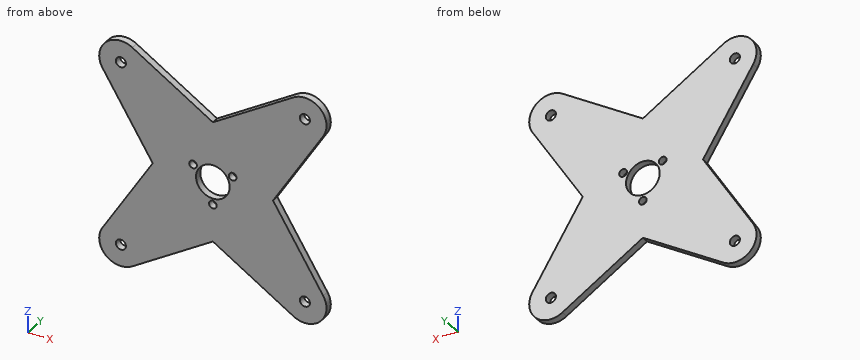
```python
from build123d import *

# Parameters (mm, degrees)
SKETCH_1_R          = 2.1
EXTRUDE_1_DEPTH     = 3
SKETCH_2_R          = 7
SKETCH_2_R_2        = 1.6
CUT_EXTRUDE_1_DEPTH = 10


with BuildPart() as part:
    # 草图1 → 凸台-拉伸1 (new body)
    with BuildSketch(Plane(origin=(0, 0, 0), x_dir=(1, 0, 0), z_dir=(0, 1, 0))):
        with BuildLine():
            Line((-45.88639118, 33.487067107), (-25, 0))
            Line((-25, 0), (-45.88639118, -33.487067107))
            ThreePointArc((-45.88639118, -33.487067107), (-44.613961031, -44.613961031), (-33.487067107, -45.88639118))
            Line((-33.487067107, -45.88639118), (0, -25))
            Line((0, -25), (33.487067107, -45.88639118))
            ThreePointArc((33.487067107, -45.88639118), (44.613961031, -44.613961031), (45.88639118, -33.487067107))
            Line((45.88639118, -33.487067107), (25, 0))
            Line((25, 0), (45.88639118, 33.487067107))
            ThreePointArc((45.88639118, 33.487067107), (44.613961031, 44.613961031), (33.487067107, 45.88639118))
            Line((33.487067107, 45.88639118), (0, 25))
            Line((0, 25), (-33.487067107, 45.88639118))
            ThreePointArc((-33.487067107, 45.88639118), (-44.613961031, 44.613961031), (-45.88639118, 33.487067107))
        make_face()
        with Locations(Location((38.25, 38.25, 0), (0, 0, 270))):
            Circle(SKETCH_1_R, mode=Mode.SUBTRACT)
        with Locations(Location((-38.25, -38.25, 0), (0, 0, 270))):
            Circle(SKETCH_1_R, mode=Mode.SUBTRACT)
        with Locations(Location((38.25, -38.25, 0), (0, 0, 270))):
            Circle(SKETCH_1_R, mode=Mode.SUBTRACT)
        with Locations(Location((-38.25, 38.25, 0), (0, 0, 270))):
            Circle(SKETCH_1_R, mode=Mode.SUBTRACT)
    extrude(amount=EXTRUDE_1_DEPTH)

    # 草图2 → 切除-拉伸1 (cut)
    with BuildSketch(Plane(origin=(0, 3, 0), x_dir=(1, 0, 0), z_dir=(0, 1, 0))):
        with Locations(Location((0, 0, 0), (0, 0, 270))):
            Circle(SKETCH_2_R)
        with Locations(Location((0, 9.5, 0), (0, 0, 270))):
            Circle(SKETCH_2_R_2)
        with Locations(Location((8.227241336, -4.75, 0), (0, 0, 270))):
            Circle(SKETCH_2_R_2)
        with Locations(Location((-8.227241336, -4.75, 0), (0, 0, 270))):
            Circle(SKETCH_2_R_2)
    extrude(amount=-CUT_EXTRUDE_1_DEPTH, mode=Mode.SUBTRACT)


solid = part.part
```
Here's how the part is built. I have some questions about the finished solid (model axes, mm). Round coordinates to 2 decimals unless told otherwise and drop trailing zeros. Write each loop counter-clockwise with the first axis right and the second up, starting at its lowest first coordinate (ties: lowest second). Pieces come first, ordered by that corner, then holes.
Q1. If we section it at C-C on z = -9.5: Write out the boundary of the cut face in (x, y), plus the area to 3 significant figures.
Q2. If we section it at A-A on z = 38.25: Write out the boundary of the cut face in (x, y).
Q3. If we section it at B-B on y = 1.2: Give the number of separate pieces and of enclosed holes in the cut face, plus the area to 3 significant figures.
Q4. If we section it at D-D on x = -38.25: Write out the boundary of the cut face in (y, z), plus the area to 3 significant figures.
Q5. Please list where these lines run through material, in increasing order: probe 1 along X at (y, z) = (1.2, 4.75); probe 2 along Z at (x, y) = (38, 2.8); probe 3 along Z at (x, y) = (-25.5, 0.25).
Q6. Will these pins go through, and if not, where does the flat tip stop? P1, Ø3.5, axis at x = 0, z = -9.5, coming from the +Y side; P2, Ø11, axis at x = 0, z = 0, coming from the -Y side.
Answer below:
1. outline: (-30.93, 0) - (-1.6, 0) - (-1.6, 3) - (-30.93, 3) - close; (1.6, 0) - (30.93, 0) - (30.93, 3) - (1.6, 3) - close
1. area: 176 mm2
2. outline: (-47.25, 0) - (-40.35, 0) - (-40.35, 3) - (-47.25, 3) - close; (-36.15, 0) - (-21.24, 0) - (-21.24, 3) - (-36.15, 3) - close; (21.24, 0) - (36.15, 0) - (36.15, 3) - (21.24, 3) - close; (40.35, 0) - (47.25, 0) - (47.25, 3) - (40.35, 3) - close
3. separate pieces: 1
3. enclosed holes: 8
3. area: 5,450 mm2
4. outline: (0, -47.25) - (3, -47.25) - (3, -40.35) - (0, -40.35) - close; (0, -36.15) - (3, -36.15) - (3, -21.24) - (0, -21.24) - close; (0, 21.24) - (3, 21.24) - (3, 36.15) - (0, 36.15) - close; (0, 40.35) - (3, 40.35) - (3, 47.25) - (0, 47.25) - close
4. area: 131 mm2
5. probe 1: x = -27.96 to -9.83, -6.63 to -5.14, 5.14 to 6.63, 9.83 to 27.96
5. probe 2: z = -47.25 to -40.34, -36.16 to -20.84, 20.84 to 36.16, 40.34 to 47.25
5. probe 3: z = -40.9 to -0.8, 0.8 to 40.9
6. P1: stops at y = 3
6. P2: passes through
